from build123d import *

# Parameters (mm, degrees)
SKETCH4_W                    = 25
SKETCH4_H                    = 50
BASE_FLANGE1_DEPTH           = 1.2
EDGE_FLANGE1_STRIP_W         = 6.2732
EDGE_FLANGE1_STRIP_H         = 1.2
EDGE_FLANGE1_STRIP_CUT_DEPTH = 50
EDGE_FLANGE1_DEPTH           = 50


# Sheet-metal steps are written as plain solids
with BuildPart() as part:
    # Sketch4 → Base-Flange1 (new body)
    with BuildSketch(Plane.XY):
        with Locations((12.5, 25)):
            Rectangle(SKETCH4_W, SKETCH4_H)
    extrude(amount=-BASE_FLANGE1_DEPTH)

    # Edge-Flange1 strip (across the edge) → Edge-Flange1 strip cut (cut)
    with BuildSketch(Plane(origin=(25, 50, -1.2), x_dir=(-1, 0, 0), z_dir=(0, -1, 0))):
        with Locations((-1.2, -0.6)):
            Rectangle(EDGE_FLANGE1_STRIP_W, EDGE_FLANGE1_STRIP_H)
    extrude(amount=EDGE_FLANGE1_STRIP_CUT_DEPTH, mode=Mode.SUBTRACT)

    # Edge-Flange1 section (across the edge) → Edge-Flange1 (add)
    with BuildSketch(Plane(origin=(25, 50, -1.2), x_dir=(-1, 0, 0), z_dir=(0, -1, 0))):
        with BuildLine():
            Line((0, 0.7366), (0, 18.8))
            Line((0, 18.8), (1.2, 18.8))
            Line((1.2, 18.8), (1.2, 0.7366))
            ThreePointArc((1.2, 0.7366), (1.415745145, 0.215745145), (1.9366, 0))
            Line((1.9366, 0), (1.9366, -1.2))
            ThreePointArc((1.9366, -1.2), (0.567217008, -0.632782992), (0, 0.7366))
        make_face()
    extrude(amount=EDGE_FLANGE1_DEPTH)


solid = part.part
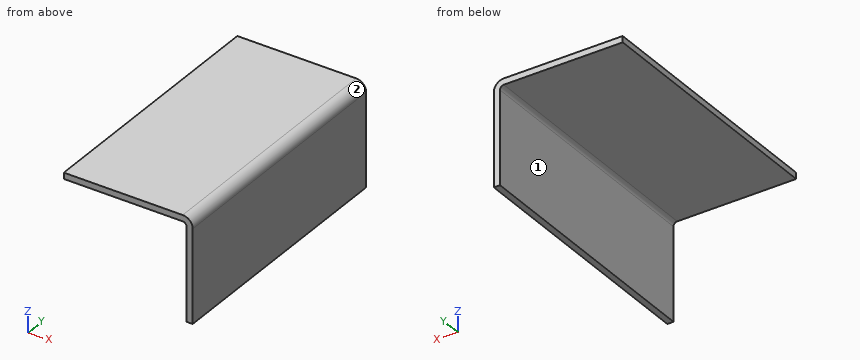
Read the model definition and answer for the solid it produces. Units are mm, in the model's axes. Face numbers are marked on the shaded views. A direction names the side the tool comes from. Round coordinates to 2 decimals unless told otherwise and drop trailing zeros. Loops run counter-clockwise (first coordinate to the right, second up) from the corner with the lowest first, then second, coordinate; pieces in that order, holes last. Notation, with made-up numbers: (81.25, -30) - (101.25, -30) arc R24 cw to (101.25, -14) - close; hole circle Ø1 at (58.5, 17.25). An arc over 180 degrees is marked (long way). One line per question, with ' | ' between items. Start each with the question number.
Q1. For the marked faces 1 and 2, determine the directions among +Z, -Z, +X, -X, +Y, -Y from which every point of the face is accessible in a straight line to the end or side of a thin tool.
Q2. Find the intervals of material crossed by L1, parallel to X at y = 11, z = -11; L2, parallel to Z at x = 7.25, y = 10.5, in increasing order.
Q3. Section C-C on z = -17.25 is taken. Give the vertices of the cut face in (x, y).
Q4. Flat-ended cylindrical pins translate along their axes: pin 1 (12 mm diameter, centred on x = 18, z = -12, fed in from -Y); pin 2 (8 mm diameter, centred on x = 4, z = -9, fed in from -Y); pin 3 (4 mm diameter, centred on y = 5.5, z = -18, fed in from -X); pin 4 (1 mm diameter, centred on x = 14, y = 16, fed in from -Z). Find the tip coordinate at first contact, or state that the pin passes through.
Q5. Section B-B on x = 3.5 is taken. Give the vertices of the cut face in (y, z).
Q6. Section A-A on y = 22 is taken. Give the vertices of the cut face in (x, z), plus the area to 3 significant figures.
Established:
1) face 1: -Z, -X, +Y, -Y | face 2: +Z, +X, +Y, -Y
2) L1: 23.8 to 25 | L2: -1.2 to 0
3) outline: (23.8, 0) - (25, 0) - (25, 50) - (23.8, 50) - close
4) pin 1: y = 0 | pin 2: through | pin 3: x = 23.8 | pin 4: z = -1.2
5) outline: (0, -1.2) - (50, -1.2) - (50, 0) - (0, 0) - close
6) outline: (0, -1.2) - (23.06, -1.2) arc R0.74 cw to (23.8, -1.94) - (23.8, -20) - (25, -20) - (25, -1.94) arc R1.94 ccw to (23.06, 0) - (0, 0) - close | area: 51.9 mm²
